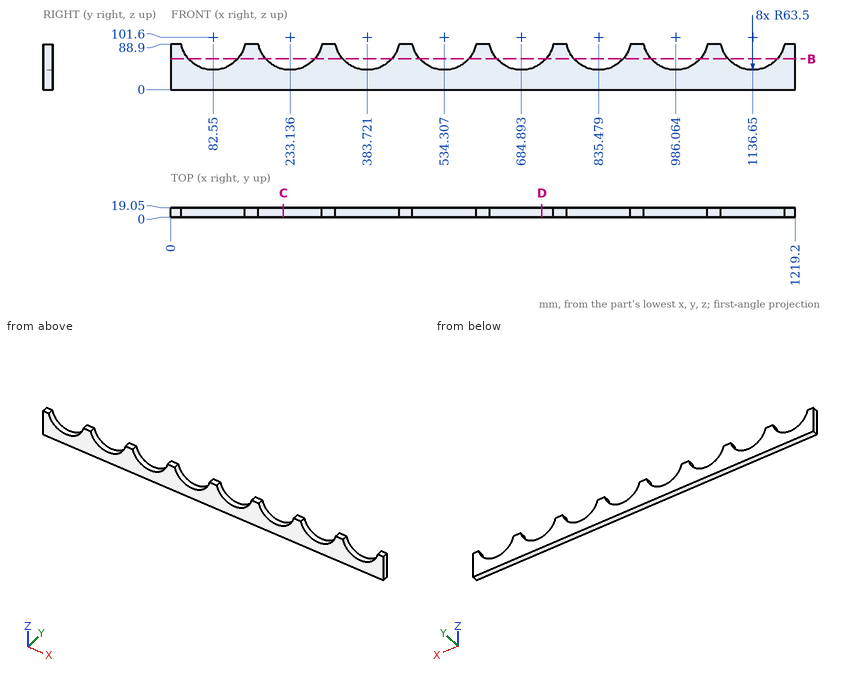
For this review, use the dimensioned drawing (mm, ordinates from the lowest corner) and the shaded views. Coordinates: 2 decimals unless noted, no trailing zeros. Write each loop counter-clockwise with the first axis right and the second up, starting at its lowest first coordinate (ties: lowest second). Pieces come first, ordered by that corner, then holes. Notation, with made-up numbers: (84.5, 75.25) -> (123.5, 75.25) arc R23 ccw to (123.5, 88.25) -> close; hole circle Ø5 at (58, 33.5). An arc over 180 degrees is marked (long way). Put each result on its own line as item: value.
Q1. Take a section at D-D, the plane x = 725. State the section outline as (y, z) points.
From the geometry:
outline: (0, 0) -> (19.05, 0) -> (19.05, 52.37) -> (0, 52.37) -> close
Q2. Take a section at B-B, the plane z = 60. Count the separate pieces of the cut face and the enclosed holes in it, then the cut area to 3 significant figures.
From the geometry:
separate pieces: 9
enclosed holes: 0
area: 8,600 mm2
Q3. Take a section at C-C, the plane x = 220. State the section outline as (y, z) points.
From the geometry:
outline: (0, 0) -> (19.05, 0) -> (19.05, 39.47) -> (0, 39.47) -> close
Q4. Wall thickness on L1, parallel to Z at x = 230, y = 6.5; L2, parallel to Z at x = 1139, y = 18.25: over which ranges is each line inside the solid? List them lowest first.
From the geometry:
L1: z = 0 to 38.18
L2: z = 0 to 38.14
